Answer from the drawing. Dimensions are ordinates in mm from the lowest x, y and z of the part. Coordinates: 2 decimals unless noted, no trailing zeros. Order: outer loops, then holes, each group sorted by start corner. A loop starts at its lowest first (then second) coordinate and runs counter-clockwise, first axis right, second up. Notation, with made-up numbers: (-4, -3.5) - (45, -3.5) arc R29 ccw to (45, 22.5) - close; hole circle Ø1 at (68, -30.5). An arc over 180 degrees is marked (long way). Answer as a JSON object with one key per item and string values. Group by question number.
1) Section B-B (z = 25) is taken. Give the vertices of the cut face in (x, y).
2) The mould has two halves that part along X. Classify the marked faces 1, 2 and 3: released by +X, released by -X, zero draft, split by the parting line, or undercut.
3) This flat-tipped pin is pushed along its axis until it touches: P1, Ø5, axis at x = 37.5, z = 27.5, coming from the -Y side. Where does it stop, or does it pass through?
4) Section A-A (x = 25) is taken. Give the vertices of the cut face in (y, z), plus the area to 3 significant figures.
5) Section C-C (y = 15.75) is taken. Give the vertices of the cut face in (x, z).
6) Find the intervals of material crossed by line 1 along X through (y, z) = (15, 25); line 2 along Z through (x, y) = (23, 5.5); line 3 along X through (y, z) = (12.25, 30), in increasing order.
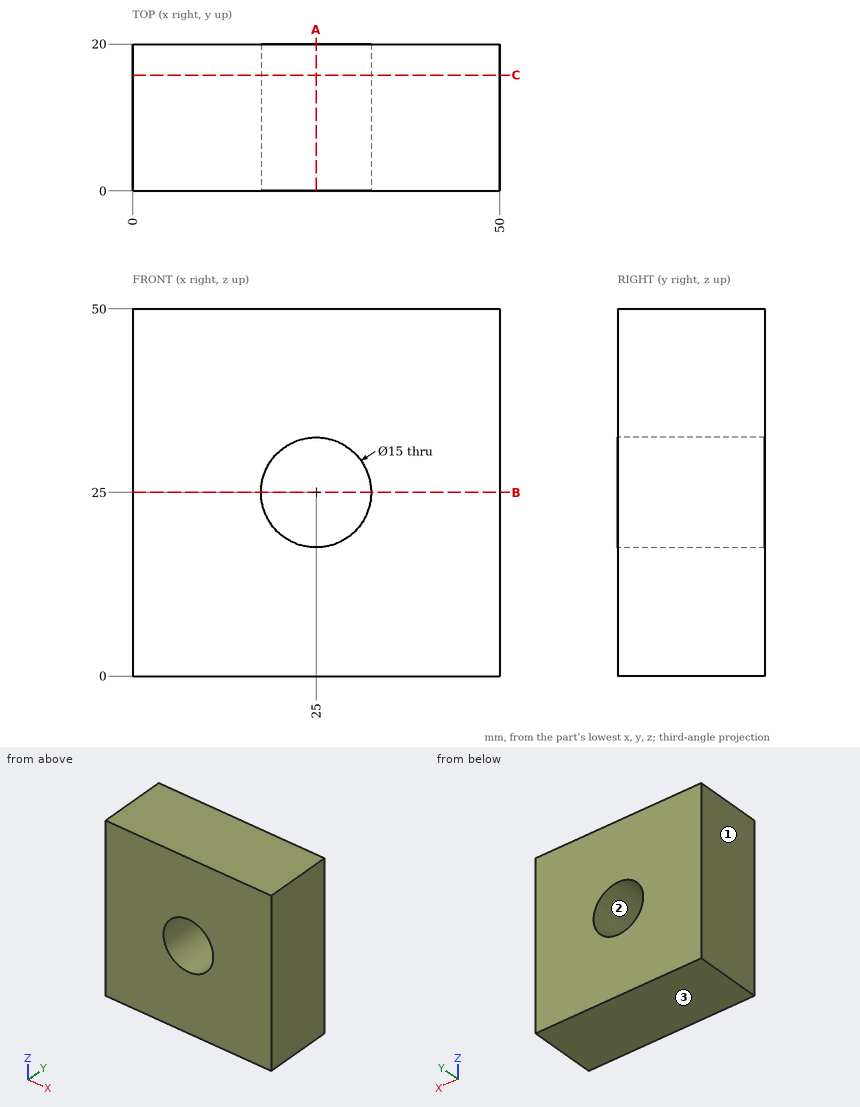
Report:
{
 "1": {"outline": "(0, 0) - (17.5, 0) - (17.5, 20) - (0, 20) - close; (32.5, 0) - (50, 0) - (50, 20) - (32.5, 20) - close"},
 "2": {"face 1": "released by -X", "face 2": "undercut", "face 3": "zero draft"},
 "3": {"P1": "stops at y = 0"},
 "4": {"outline": "(0, 0) - (20, 0) - (20, 17.5) - (0, 17.5) - close; (0, 32.5) - (20, 32.5) - (20, 50) - (0, 50) - close", "area": "700 mm²"},
 "5": {"outline": "(0, 0) - (50, 0) - (50, 50) - (0, 50) - close; hole circle Ø15 at (25, 25)"},
 "6": {"line 1": "x = 0 to 17.5, 32.5 to 50", "line 2": "z = 0 to 17.77, 32.23 to 50", "line 3": "x = 0 to 19.41, 30.59 to 50"}
}
